Source: CAD feature listing. Evaluate the final solid. Frame: model axes, mm. A direction names the side the tool comes from. Round coordinates to 2 decimals unless told otherwise and drop trailing zeros. Order: outer loops, then holes, each group sorted by start corner. A loop starts at its lowest first (then second) coordinate and runs counter-clockwise, first axis right, second up. Notation, with made-up numbers: M 21.5,-21 L 32.5,-21 A28 cw 32.5,6 Z; hole C 30,59.25 d8. An arc over 180 degrees is marked long. Answer in a Markdown table with one row per item. Add a question column.
```python
from build123d import *

# Parameters (mm, degrees)
MODEL_R                 = 1.5
SALIENTE_EXTRUIR1_DEPTH = 3


with BuildPart() as part:
    # Model → Saliente-Extruir1 (new body)
    with BuildSketch(Plane.XY):
        with BuildLine():
            Line((160.698926217, 226.370073483), (160.698926217, 239.515886932))
            ThreePointArc((160.698926217, 239.515886932), (159.517719337, 242.924264089), (156.212886551, 244.370073483))
            Line((156.212886551, 244.370073483), (147.202886551, 244.370073483))
            ThreePointArc((147.202886551, 244.370073483), (142.702886551, 239.870073483), (147.202886551, 235.370073483))
            Line((147.202886551, 235.370073483), (151.698926217, 235.370073483))
            Line((151.698926217, 235.370073483), (151.698926217, 226.370073483))
            ThreePointArc((151.698926217, 226.370073483), (156.198926217, 221.870073483), (160.698926217, 226.370073483))
        make_face()
        with Locations((156.198926217, 226.370073483)):
            Circle(MODEL_R, mode=Mode.SUBTRACT)
        with BuildLine():
            ThreePointArc((147.087886551, 238.370073483), (145.587886551, 239.870073483), (147.087886551, 241.370073483))
            Line((147.087886551, 241.370073483), (156.212886551, 241.370073483))
            ThreePointArc((156.212886551, 241.370073483), (157.712886551, 239.870073483), (156.212886551, 238.370073483))
            Line((156.212886551, 238.370073483), (147.087886551, 238.370073483))
        make_face(mode=Mode.SUBTRACT)
    extrude(amount=SALIENTE_EXTRUIR1_DEPTH)


solid = part.part
```
(1) Cut plane A-A (x = 148.25). Return loops of the section in (y, z).
(2) Draft query along X for faces 1 (the face through (159.55, 242.89, 1.48)), 2 (the face through (154, 236, 3)), 3 (the face through (157.585, 225.796, 1.479)), 4 (the face through (157.713, 239.903, 1.479)). Return one class per face: +X half, -X half, draft (parallel to the pull), parting line (faces both ways), or undercut.
(3) Line query: line 1 (Y direction, x = 156, z = 2.8); line 2 (Y direction, x = 157, z = 0.55); line 3 (Y direction, x = 148.25, z = 2.15). Output: solid intervals per line, ascending. Write a range as from..to.
(4) Cut plane D-D (y = 234). Return loops of the section in (x, z).
(5) Cut plane C-C (y = 226). Return loops of the section in (x, z), and give its area (3 significant figures).
(6) Pin query (flat end, axial travel): pin 1 (2 mm diameter, centred on x = 156, y = 226, fed in from -Z); pin 2 (1.5 mm diameter, centred on y = 229, z = 1.5, fed in from -X); pin 3 (0.9 mm diameter, centred on x = 153.5, z = 1.5, fed in from -Y); pin 4 (1 mm diameter, centred on y = 237.5, z = 2.5, fed in from +X). Return the tip coordinate at first contact, or that it passes through.
(7) Access query for faces 5 (the face through (154, 236, 0)), 6 (the face through (152, 241.37, 1)), 7 (the face through (151.699, 231, 1)). Directions: +Z, -Z, +X, -X, +Y, -Y. A direction counts if a zero-diameter tool reaches every point of the face in a straight line with its end or side. Return the directions, or none.
(8) Cut plane B-B (z = 0.5). Return loops of the section in (x, y), and give its area (3 significant figures).
Answer list:
| question | item | result |
|---|---|---|
| 1 | outline | M 235.37,0 L 238.37,0 L 238.37,3 L 235.37,3 Z; M 241.37,0 L 244.37,0 L 244.37,3 L 241.37,3 Z |
| 2 | face 1 | +X half |
| 2 | face 2 | draft |
| 2 | face 3 | undercut |
| 2 | face 4 | undercut |
| 3 | line 1 | 221.87..224.88, 227.86..238.37, 241.37..244.37 |
| 3 | line 2 | 221.94..225.1, 227.64..238.59, 241.15..244.3 |
| 3 | line 3 | 235.37..238.37, 241.37..244.37 |
| 4 | outline | M 151.7,0 L 160.7,0 L 160.7,3 L 151.7,3 Z |
| 5 | outline | M 151.71,0 L 154.75,0 L 154.75,3 L 151.71,3 Z; M 157.65,0 L 160.68,0 L 160.68,3 L 157.65,3 Z |
| 5 | area | 18.2 mm² |
| 6 | pin 1 | through |
| 6 | pin 2 | x = 151.7 |
| 6 | pin 3 | y = 222.47 |
| 6 | pin 4 | x = 160.7 |
| 7 | face 5 | -Z, +X, -X, +Y, -Y |
| 7 | face 6 | +Z, -Z |
| 7 | face 7 | +Z, -Z, -X, -Y |
| 8 | outline | M 147.2,235.37 L 151.7,235.37 L 151.7,226.37 A4.5 ccw 160.7,226.37 L 160.7,239.52 A4.5 ccw 156.21,244.37 L 147.2,244.37 A4.5 ccw Z; hole M 147.09,238.37 L 156.21,238.37 A1.5 ccw 156.21,241.37 L 147.09,241.37 A1.5 ccw Z; hole C 156.2,226.37 d3 |
| 8 | area | 220 mm² |
